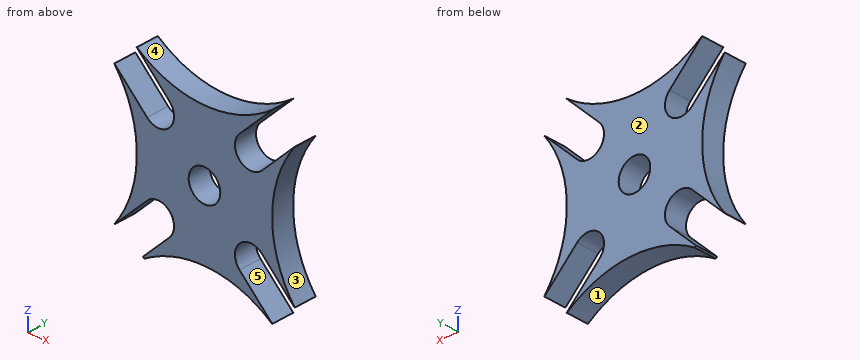
```python
from build123d import *

# Parameters (mm, degrees)
F0_R     = 3.5
F1_DEPTH = 5


with BuildPart() as f1:
    # F0 (on Front) → F1 (new body)
    with BuildSketch(Plane.XZ):
        with BuildLine():
            ThreePointArc((-56.449953, 26.068207), (-42.088166, 29.926809), (-28.075866, 24.946327))
            ThreePointArc((-28.075866, 24.946327), (-28.061514, 24.9571), (-28.047169, 24.967882))
            Line((-28.047169, 24.967882), (-35.297692, 32.218405))
            Line((-35.297692, 32.218405), (-43.075866, 39.99658))
            Line((-43.075866, 39.99658), (-50.854041, 32.218405))
            Line((-50.854041, 32.218405), (-56.704745, 26.367701))
            Line((-56.704745, 26.367701), (-56.449953, 26.068207))
        make_face()
        with BuildLine():
            Line((-43.075866, 39.99658), (-35.297692, 32.218405))
            ThreePointArc((-35.297692, 32.218405), (-35.297692, 37.168153), (-30.347944, 37.168153))
            Line((-30.347944, 37.168153), (-38.126119, 44.946327))
            Line((-38.126119, 44.946327), (-30.347944, 52.724502))
            ThreePointArc((-30.347944, 52.724502), (-35.297692, 52.724502), (-35.297692, 57.674249))
            Line((-35.297692, 57.674249), (-43.075866, 49.896075))
            Line((-43.075866, 49.896075), (-50.854041, 57.674249))
            ThreePointArc((-50.854041, 57.674249), (-50.854041, 52.724502), (-55.803788, 52.724502))
            Line((-55.803788, 52.724502), (-48.025614, 44.946327))
            Line((-48.025614, 44.946327), (-55.803788, 37.168153))
            ThreePointArc((-55.803788, 37.168153), (-50.854041, 37.168153), (-50.854041, 32.218405))
            Line((-50.854041, 32.218405), (-43.075866, 39.99658))
        make_face()
        with Locations((-43.075866, 44.946327)):
            Circle(F0_R, mode=Mode.SUBTRACT)
        with BuildLine():
            Line((-30.347944, 37.168153), (-23.097422, 29.91763))
            ThreePointArc((-23.097422, 29.91763), (-23.086639, 29.931975), (-23.075866, 29.946327))
            ThreePointArc((-23.075866, 29.946327), (-28.075866, 44.946327), (-23.075866, 59.946327))
            ThreePointArc((-23.075866, 59.946327), (-23.086639, 59.96068), (-23.097422, 59.975025))
            Line((-23.097422, 59.975025), (-30.347944, 52.724502))
            Line((-30.347944, 52.724502), (-38.126119, 44.946327))
            Line((-38.126119, 44.946327), (-30.347944, 37.168153))
        make_face()
        with BuildLine():
            Line((-63.054311, 29.91763), (-55.803788, 37.168153))
            Line((-55.803788, 37.168153), (-48.025614, 44.946327))
            Line((-48.025614, 44.946327), (-55.803788, 52.724502))
            Line((-55.803788, 52.724502), (-63.054311, 59.975025))
            ThreePointArc((-63.054311, 59.975025), (-63.065094, 59.96068), (-63.075866, 59.946327))
            ThreePointArc((-63.075866, 59.946327), (-58.075866, 44.946327), (-63.075866, 29.946327))
            ThreePointArc((-63.075866, 29.946327), (-63.065094, 29.931975), (-63.054311, 29.91763))
        make_face()
        with BuildLine():
            Line((-43.075866, 49.896075), (-35.297692, 57.674249))
            Line((-35.297692, 57.674249), (-28.047169, 64.924772))
            ThreePointArc((-28.047169, 64.924772), (-28.061514, 64.935555), (-28.075866, 64.946327))
            ThreePointArc((-28.075866, 64.946327), (-43.075866, 59.946327), (-58.075866, 64.946327))
            ThreePointArc((-58.075866, 64.946327), (-58.090219, 64.935555), (-58.104564, 64.924772))
            Line((-58.104564, 64.924772), (-50.854041, 57.674249))
            Line((-50.854041, 57.674249), (-43.075866, 49.896075))
        make_face()
    extrude(amount=F1_DEPTH)


solid = f1.part
```
Can you work these out from the model? Positions are in its coordinate system, mm. Face numbers are marked on the shaded views. A direction names the side the tool comes from. Coordinates: 2 decimals unless noted, no trailing zeros. Loops run counter-clockwise (first coordinate to the right, second up) from the corner with the lowest first, then second, coordinate; pieces in that order, holes last.
1) For pin 1 (1.5 mm diameter, centred on x = -51.5, y = -2, fed in from -Z); pin 2 (3 mm diameter, centred on y = -0.5, z = 39, fed in from -X), each with a flat end and sliding along its axis, tell me the tip position at first contact or that it passes through.
2) Imagine slicing it at A-A on z = 57. List the corners of the cut face in (x, y) for me.
3) Thinking about a two-plate mould opening in X: for the marked faces 1, 2 and 3, which applies, pulls with the +X half, pulls with the -X half, needs draft (parallel to the pull), parting line crosses it, or undercut?
4) Imagine slicing it at D-D on z = 44. List the corners of the cut face in (x, y) for me.
5) Imagine slicing it at B-B on x = -54.5. List the corners of the cut face in (y, z) for me, plus the area to 3 significant figures.
6) Which directions (+Z, -Z, +X, -X, +Y, -Y) give clear straight access to the entire face, cutting with the end or side of a thin tool? Please do the marked faces 4 and 5.
7) Imagine slicing it at C-C on x = -44.5. List the corners of the cut face in (y, z) for me.
8) I need wall thicknesses on probe 1 along X at (y, z) = (-3.3, 54); probe 2 along Z at (x, y) = (-55, -2.95); probe 3 along X at (y, z) = (-1.95, 57). Which ranges of each line are inside material? Lowest first, please.
Completed:
1. pin 1: stops at z = 28.2
1. pin 2: stops at x = -59.21
2. outline: (-61.17, -5) - (-60.08, -5) - (-60.08, 0) - (-61.17, 0) - close; (-50.33, -5) - (-35.82, -5) - (-35.82, 0) - (-50.33, 0) - close; (-26.07, -5) - (-24.98, -5) - (-24.98, 0) - (-26.07, 0) - close
3. face 1: undercut
3. face 2: needs draft
3. face 3: pulls with the +X half
4. outline: (-58.09, -5) - (-46.45, -5) - (-46.45, 0) - (-58.09, 0) - close; (-39.71, -5) - (-28.06, -5) - (-28.06, 0) - (-39.71, 0) - close
5. outline: (-5, 27.18) - (0, 27.18) - (0, 28.57) - (-5, 28.57) - close; (-5, 37.99) - (0, 37.99) - (0, 51.9) - (-5, 51.9) - close; (-5, 61.32) - (0, 61.32) - (0, 62.71) - (-5, 62.71) - close
5. area: 83.4 mm2
6. face 4: +Z, +Y, -Y
6. face 5: +Y, -Y
7. outline: (-5, 29.91) - (0, 29.91) - (0, 41.75) - (-5, 41.75) - close; (-5, 48.14) - (0, 48.14) - (0, 59.99) - (-5, 59.99) - close
8. probe 1: x = -59.77 to -57.08, -50.04 to -36.11, -29.07 to -26.38
8. probe 2: z = 26.92 to 28.07, 37.77 to 52.12, 61.82 to 62.97
8. probe 3: x = -61.17 to -60.08, -50.33 to -35.82, -26.07 to -24.98
